Model file for the job. Use its own axes, mm. Face numbers are marked on the shaded views. A direction names the side the tool comes from. Give positions to 0.01 mm unless a question says otherwise; leave off trailing zeros. Loops run counter-clockwise (first coordinate to the right, second up) from the corner with the lowest first, then second, coordinate; pieces in that order, holes last. Notation, with made-up numbers: M 23.5,8.5 L 39.5,8.5 A4 ccw 39.5,12.5 Z; hole C 14.25,47.5 d11. An arc over 180 degrees is marked long. Answer in a Markdown table with one row per item.
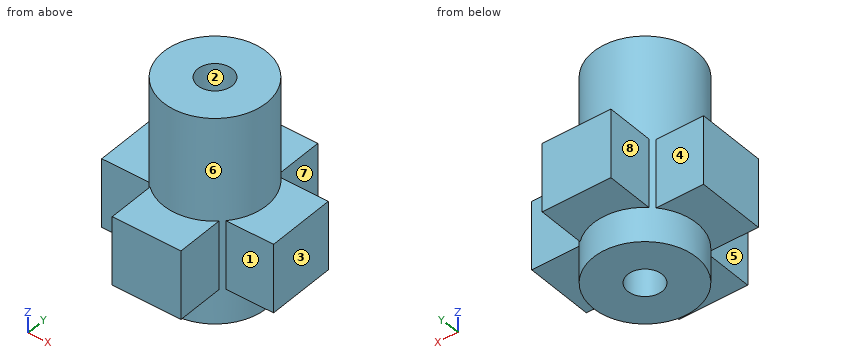
```python
from build123d import *

# Parameters (mm, degrees)
SKETCH1_R                = 7.5
SKETCH1_R_2              = 2.5
BOSS_EXTRUDE1_DEPTH      = 10
BOSS_EXTRUDE2_DEPTH      = 15
BOSS_EXTRUDE2_DEPTH_BACK = 15
SKETCH2_R                = 7.5
SKETCH2_R_2              = 2.5


with BuildPart() as part:
    # Sketch1 → Boss-Extrude1 (new body)
    # profile 1 of 5: a face of its own
    with BuildSketch(Plane.XY):
        with BuildLine():
            Line((-12.5, -5), (-5.590169944, -5))
            ThreePointArc((-5.590169944, -5), (-7.5, 0), (-5.590169944, 5))
            Line((-5.590169944, 5), (-12.5, 5))
            Line((-12.5, 5), (-12.5, -5))
        make_face()
    # profile 2 of 5: a face of its own
    with BuildSketch(Plane.XY):
        with BuildLine():
            ThreePointArc((5, -5.590169944), (0, -7.5), (-5, -5.590169944))
            Line((-5, -5.590169944), (-5, -12.5))
            Line((-5, -12.5), (5, -12.5))
            Line((5, -12.5), (5, -5.590169944))
        make_face()
    # profile 3 of 5: a face of its own
    with BuildSketch(Plane.XY):
        with BuildLine():
            Line((-5, 12.5), (-5, 5.590169944))
            ThreePointArc((-5, 5.590169944), (0, 7.5), (5, 5.590169944))
            Line((5, 5.590169944), (5, 12.5))
            Line((5, 12.5), (-5, 12.5))
        make_face()
    # profile 4 of 5: a face of its own
    with BuildSketch(Plane.XY):
        with BuildLine():
            ThreePointArc((7.5, 0), (7.006292692, -2.676165673), (5.590169944, -5))
            Line((5.590169944, -5), (12.5, -5))
            Line((12.5, -5), (12.5, 5))
            Line((12.5, 5), (5.590169944, 5))
            ThreePointArc((5.590169944, 5), (7.006292692, 2.676165673), (7.5, 0))
        make_face()
    # profile 5 of 5: a face of its own
    with BuildSketch(Plane.XY):
        Circle(SKETCH1_R)
        Circle(SKETCH1_R_2, mode=Mode.SUBTRACT)
    extrude(amount=BOSS_EXTRUDE1_DEPTH)

    # Sketch2 → Boss-Extrude2 (add, two sides: drawn at the far end of the back side and taken through both)
    with BuildSketch(Plane.XY.offset(10).offset(-BOSS_EXTRUDE2_DEPTH_BACK)):
        Circle(SKETCH2_R)
        Circle(SKETCH2_R_2, mode=Mode.SUBTRACT)
    extrude(amount=BOSS_EXTRUDE2_DEPTH + BOSS_EXTRUDE2_DEPTH_BACK)


solid = part.part
```
(1) Saw through at D-D, the plane x = -4.5. Give the cut face in (y, z).
Established:
| item | result |
|---|---|
| outline | M -12.5,0 L -6,0 L -6,-5 L 6,-5 L 6,0 L 12.5,0 L 12.5,10 L 6,10 L 6,25 L -6,25 L -6,10 L -12.5,10 Z |
(2) Wall check: L1, parallel to Y at x = 0, z = 4.5; L2, parallel to X at y = -8.5, z = 8; L3, parallel to X at y = -0.75, z = 14.75. Give the ranges that are in metal, low to high.
Established:
| item | result |
|---|---|
| L1 | y = -12.5 to -2.5, 2.5 to 12.5 |
| L2 | x = -5 to 5 |
| L3 | x = -7.46 to -2.38, 2.38 to 7.46 |
(3) Flat gauge pins, fed straight in: P1, Ø5.5, axis at x = 9, z = 7, coming from the -Y side; P2, Ø5.5, axis at x = 8, z = 6.5, coming from the +Y side; P3, Ø3, axis at y = -1.5, z = 20.5, coming from the +X side; P4, Ø4, axis at x = 0, y = 0, coming from the +Z side. Where does each tip first touch, or does it go through?
Established:
| item | result |
|---|---|
| P1 | stops at y = -5 |
| P2 | stops at y = 5.36 |
| P3 | stops at x = 7.5 |
| P4 | passes through |
(4) Mould opens along Y. For the marked faces 1, 2, 3 and 4 say: pulls with the +Y half, pulls with the -Y half, needs draft (parallel to the pull), parting line crosses it, or undercut.
Established:
| item | result |
|---|---|
| face 1 | pulls with the -Y half |
| face 2 | undercut |
| face 3 | needs draft |
| face 4 | pulls with the +Y half |
(5) Saw through at A-A, the plane x = 0. Give the cut face in (y, z).
Established:
| item | result |
|---|---|
| outline | M -12.5,0 L -7.5,0 L -7.5,-5 L -2.5,-5 L -2.5,25 L -7.5,25 L -7.5,10 L -12.5,10 Z; M 2.5,-5 L 7.5,-5 L 7.5,0 L 12.5,0 L 12.5,10 L 7.5,10 L 7.5,25 L 2.5,25 Z |
(6) Which spindle directions (+Z, -Z, +X, -X, +Y, -Y) get a long thin tool onto all of the face, cutting with end or side? Do the marked faces 5, 6, 7 and 8. Say none if no direction does.
Established:
| item | result |
|---|---|
| face 5 | +Z, -Z, -X, -Y |
| face 6 | none |
| face 7 | +Z, -Z, +X, +Y |
| face 8 | +Z, -Z, -X, +Y |
(7) Saw through at C-C, the plane z = 3.5. Give the cut face in (x, y).
Established:
| item | result |
|---|---|
| outline | M -12.5,-5 L -5.59,-5 A7.5 ccw -5,-5.59 L -5,-12.5 L 5,-12.5 L 5,-5.59 A7.5 ccw 5.59,-5 L 12.5,-5 L 12.5,5 L 5.59,5 A7.5 ccw 5,5.59 L 5,12.5 L -5,12.5 L -5,5.59 A7.5 ccw -5.59,5 L -12.5,5 Z; hole C 0,0 d5 |
